Model file for the job. Use its own axes, mm. Face numbers are marked on the shaded views. A direction names the side the tool comes from. Give positions to 0.01 mm unless a question says otherwise; leave off trailing zeros. Write each loop counter-clockwise with the first axis right and the second up, starting at its lowest first coordinate (ties: lowest second). Pieces come first, ordered by that corner, then holes.
```python
from build123d import *

# Parameters (mm, degrees)
SKETCH2_R      = 9.525
EXTRUDE1_DEPTH = 153.924
SKETCH3_R      = 14.478
EXTRUDE2_DEPTH = 5.334
FILLET1_R      = 2.54


with BuildPart() as part:
    # Sketch2 → Extrude1 (new body)
    with BuildSketch(Plane(origin=(0, 0, 0), x_dir=(1, 0, 0), z_dir=(0, 1, 0))):
        Circle(SKETCH2_R)
    extrude(amount=EXTRUDE1_DEPTH)

    # Sketch3 → Extrude2 (add)
    with BuildSketch(Plane(origin=(0, 153.924, 0), x_dir=(-1, 0, 0), z_dir=(0, 1, 0))):
        Circle(SKETCH3_R)
    extrude(amount=EXTRUDE2_DEPTH)

    # Sketch14 → Cut-Revolve1 (revolve, cut)
    with BuildSketch(Plane.XY):
        with BuildLine():
            Line((9.525, 148.463), (9.525, 142.621))
            ThreePointArc((9.525, 142.621), (7.610493481, 145.542), (9.525, 148.463))
        make_face()
    revolve(axis=Axis((0, 145.542, 0), (0, 1, 0)), mode=Mode.SUBTRACT)

    # Fillet1
    fillet1_edges = [part.edges().sort_by_distance(p)[0] for p in [
        (14.478, 159.258, 0),
    ]]
    fillet(fillet1_edges, radius=FILLET1_R)


solid = part.part
```
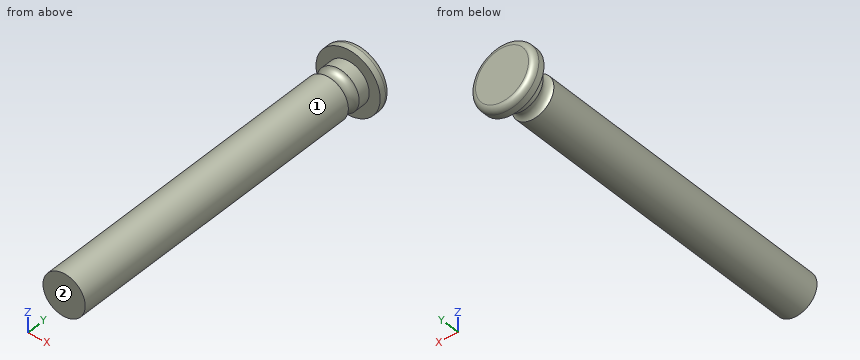
1. Slice it at C-C, the plane y = 115.5. Write the cut outline in (x, z) (3 decimals).
Calculated:
outline: circle Ø19.05 at (0, 0)
2. Probe probe 1 along X at (y, z) = (132, 0.25); probe 2 along Y at (x, z) = (-3.75, 8); probe 3 along Y at (x, z) = (6.25, -7.5). List the from-to ranges inside material, lowest first.
Calculated:
probe 1: x = -9.52 to 9.52
probe 2: y = 0 to 143.03, 148.05 to 159.26
probe 3: y = 153.92 to 159.26
3. Which spindle directions (+Z, -Z, +X, -X, +Y, -Y) get a long thin tool onto all of the face, cutting with end or side? Do the marked faces 1 and 2. Say none if no direction does.
Calculated:
face 1: -Y
face 2: +Z, -Z, +X, -X, -Y
4. Pin check, flat tips, straight feed: P1, Ø12, axis at x = -1, y = 71.5, coming from the +Z side (3 decimals); P2, Ø1, axis at x = 5, y = 41.5, coming from the -Z side (3 decimals); P3, Ø10, axis at x = -6, y = 103, coming from the -Z side. Stop position of each tip, or through.
Calculated:
P1: stops at z = 9.525
P2: stops at z = -8.395
P3: stops at z = -9.47
5. Slice it at A-A, the plane x = 0. Write the cut outline in (y, z) (3 decimals), and give its area (3 significant figures).
Calculated:
outline: (0, -9.525) - (142.621, -9.525) arc R3.186 cw to (148.463, -9.525) - (153.924, -9.525) - (153.924, -14.478) - (156.718, -14.478) arc R2.54 ccw to (159.258, -11.938) - (159.258, 11.938) arc R2.54 ccw to (156.718, 14.478) - (153.924, 14.478) - (153.924, 9.525) - (148.463, 9.525) arc R3.186 cw to (142.621, 9.525) - (0, 9.525) - close
area: 3,070 mm2
6. Slice it at B-B, the plane z = 0. Write the cut outline in (x, y) (3 decimals), and give its area (3 significant figures).
Calculated:
outline: (-14.478, 153.924) - (-9.525, 153.924) - (-9.525, 148.463) arc R3.186 cw to (-9.525, 142.621) - (-9.525, 0) - (9.525, 0) - (9.525, 142.621) arc R3.186 cw to (9.525, 148.463) - (9.525, 153.924) - (14.478, 153.924) - (14.478, 156.718) arc R2.54 ccw to (11.938, 159.258) - (-11.938, 159.258) arc R2.54 ccw to (-14.478, 156.718) - close
area: 3,070 mm2
